```python
from build123d import *

# Parameters (mm, degrees)
BOSS_EXTRUDE2_DEPTH     = 500
SKETCH3_W               = 250
SKETCH3_H               = 50
CUT_EXTRUDE1_DEPTH      = 6
SKETCH5_W               = 50
SKETCH5_H               = 25
BOSS_EXTRUDE3_DEPTH     = 5
SKETCH7_W               = 50
SKETCH7_H               = 25
BOSS_EXTRUDE4_DEPTH     = 5
SKETCH8_R               = 2.5
CUT_EXTRUDE4_DEPTH      = 256
CUT_EXTRUDE4_DEPTH_BACK = 6
SKETCH11_R              = 5
BOSS_EXTRUDE15_DEPTH    = 250
BOSS_EXTRUDE16_DEPTH    = 10
BOSS_EXTRUDE17_DEPTH    = 10
CUT_EXTRUDE5_START      = -17
SKETCH30_R              = 2.5
CUT_EXTRUDE5_DEPTH      = 306.484848098
SKETCH31_R              = 2.5
CUT_EXTRUDE6_DEPTH      = 17


with BuildPart() as part:
    # Sketch2 → Boss-Extrude2 (new body)
    with BuildSketch(Plane.XY):
        Polygon((-130, 0), (130, 0), (130, 80), (115, 80), (115, 75), (125, 75), (125, 5), (-125, 5), (-125, 75), (-115, 75), (-115, 80), (-130, 80), align=None)
    extrude(amount=BOSS_EXTRUDE2_DEPTH)

    # Sketch3 → Cut-Extrude1 (cut, through all)
    with BuildSketch(Plane(origin=(0, 5, 0), x_dir=(1, 0, 0), z_dir=(0, 1, 0))):
        with Locations((0, -475)):
            Rectangle(SKETCH3_W, SKETCH3_H)
    extrude(amount=-CUT_EXTRUDE1_DEPTH, mode=Mode.SUBTRACT)

    # Sketch5 → Boss-Extrude3 (add)
    with BuildSketch(Plane.ZY.offset(-125)):
        with Locations((475, -12.5)):
            Rectangle(SKETCH5_W, SKETCH5_H)
    extrude(amount=-BOSS_EXTRUDE3_DEPTH)

    # Sketch7 → Boss-Extrude4 (add)
    with BuildSketch(Plane(origin=(-125, 0, 0), x_dir=(0, 0, -1), z_dir=(1, 0, 0))):
        with Locations((-475, -12.5)):
            Rectangle(SKETCH7_W, SKETCH7_H)
    extrude(amount=-BOSS_EXTRUDE4_DEPTH)

    # Sketch8 → Cut-Extrude4 (cut, two sides)
    with BuildSketch(Plane.ZY.offset(-125)) as cut_extrude4_sk:
        with Locations((470, 2.5)):
            Circle(SKETCH8_R)
    extrude(amount=CUT_EXTRUDE4_DEPTH, mode=Mode.SUBTRACT)
    extrude(cut_extrude4_sk.sketch, amount=-CUT_EXTRUDE4_DEPTH_BACK, mode=Mode.SUBTRACT)

    # Sketch11 → Boss-Extrude15 (add)
    with BuildSketch(Plane.ZY.offset(-125)):
        with Locations((480, 65)):
            Circle(SKETCH11_R)
    extrude(amount=BOSS_EXTRUDE15_DEPTH)

    # Sketch27 → Boss-Extrude16 (add)
    with BuildSketch(Plane(origin=(130, 0, 0), x_dir=(0, 0, -1), z_dir=(1, 0, 0))):
        Polygon((-20, 0), (-2.121320344, -17.878679656), (-4.242640687, -20), (-24.242640687, 0), align=None)
        Polygon((-39.798989873, 0), (-12.02081528, -27.778174593), (-14.142135624, -29.899494937), (-44.04163056, 0), align=None)
    boss_extrude16 = extrude(amount=-BOSS_EXTRUDE16_DEPTH)

    # Mirror1: Boss-Extrude16 across plane
    add(boss_extrude16.mirror(Plane.ZY))

    # Sketch29 → Boss-Extrude17 (add)
    with BuildSketch(Plane(origin=(130, 0, 0), x_dir=(0, 0, -1), z_dir=(1, 0, 0))):
        Polygon((-400, 0), (-420, -20), (-417.878679656, -22.121320344), (-395.757359313, 0), align=None)
        Polygon((-380.201010127, 0), (-410.100505063, -29.899494937), (-407.97918472, -32.02081528), (-375.95836944, 0), align=None)
    boss_extrude17 = extrude(amount=-BOSS_EXTRUDE17_DEPTH)

    # Mirror2: Boss-Extrude17 across plane
    add(boss_extrude17.mirror(Plane.ZY))

    # Sketch30 → Cut-Extrude5 (cut)
    with BuildSketch(Plane(origin=(0, 187.97918472, 187.97918472), x_dir=(1, 0, 0), z_dir=(0, -0.707106781, -0.707106781)).offset(CUT_EXTRUDE5_START)):
        with Locations((125, 306.126983722)):
            Circle(SKETCH30_R)
    cut_extrude5 = extrude(amount=CUT_EXTRUDE5_DEPTH, mode=Mode.SUBTRACT)

    # Mirror3: Cut-Extrude5 across plane
    add(cut_extrude5.mirror(Plane.ZY), mode=Mode.SUBTRACT)

    # Sketch31 → Cut-Extrude6 (cut)
    with BuildSketch(Plane(origin=(0, -22.02081528, 22.02081528), x_dir=(1, 0, 0), z_dir=(0, -0.707106781, 0.707106781))):
        with Locations((125, -6.142135624)):
            Circle(SKETCH31_R)
    cut_extrude6 = extrude(amount=-CUT_EXTRUDE6_DEPTH, mode=Mode.SUBTRACT)

    # Mirror5: Cut-Extrude6 across plane
    add(cut_extrude6.mirror(Plane.ZY), mode=Mode.SUBTRACT)


solid = part.part
```
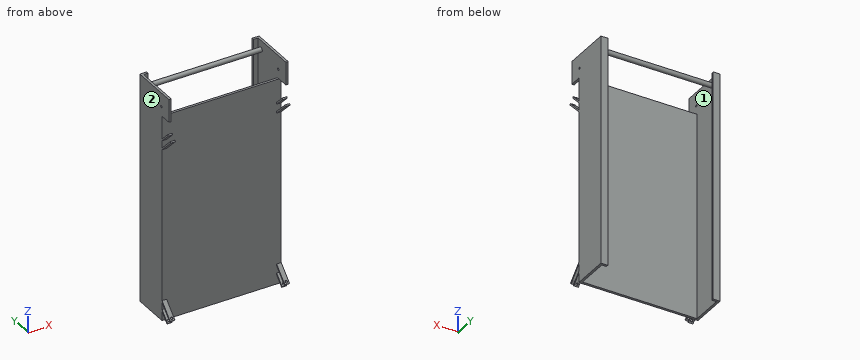
Verification items for the finished model (mm, model axes). Face numbers are marked on the shaded views. Coordinates: 2 decimals unless noted, no trailing zeros. Order: outer loops, then holes, each group sorted by start corner. A loop starts at its lowest first (then second) coordinate and runs counter-clockwise, first axis right, second up. Notation, with made-up numbers: (88.25, 40) - (145.25, 40) arc R18 cw to (145.25, 48) - close; hole circle Ø3 at (62, 52.5). An arc over 180 degrees is marked (long way). Return JSON: item names as keys, results as strings.
(1) Go/stop test with flat-tipped pins: pin 1 (16 mm diameter, centred on y = -17.5, z = 387, fed in from -X); pin 2 (4 mm diameter, centred on x = -128, z = 476.5, fed in from -Y); pin 3 (3 mm diameter, centred on x = -121, z = 282.5, fed in from -Y); pin 4 (4 mm diameter, centred on x = -127, y = -13, fed in from -Z). Record where each tip stops, or that it passes through.
Filled sheet:
{"pin 1": "stops at x = -130", "pin 2": "stops at y = -25", "pin 3": "stops at y = 0", "pin 4": "stops at z = 5.03"}
(2) Section check A-A, the plane y = 48. Record the cut outline in (x, z), and give its area (3 significant figures).
Filled sheet:
{"outline": "(-130, 0) - (-125, 0) - (-125, 500) - (-130, 500) - close; (125, 0) - (130, 0) - (130, 500) - (125, 500) - close", "area": "5,000 mm^2"}
(3) Thickness scan on line 1 along X through (y, z) = (19, 354.5); line 2 along Z through (x, y) = (127, 2); line 3 along Z through (x, y) = (-126.3, 2.5). Record the ranges inside material, lowest first.
Filled sheet:
{"line 1": "x = -130 to -125, 125 to 130", "line 2": "z = 0 to 467.55, 472.45 to 500", "line 3": "z = 0 to 467.5, 472.5 to 500"}
(4) Section check D-D, the plane z = 336. Record the cut outline in (x, y).
Filled sheet:
{"outline": "(-130, 0) - (130, 0) - (130, 80) - (115, 80) - (115, 75) - (125, 75) - (125, 5) - (-125, 5) - (-125, 75) - (-115, 75) - (-115, 80) - (-130, 80) - close"}
(5) Section check C-C, the plane z = 461. Record the cut outline in (x, y).
Filled sheet:
{"outline": "(-130, -25) - (-125, -25) - (-125, 75) - (-115, 75) - (-115, 80) - (-130, 80) - close; (115, 75) - (125, 75) - (125, -25) - (130, -25) - (130, 80) - (115, 80) - close"}
(6) Mould release check, pull along Y, two halves, no side actions. Record for the marked faces 1 and 2: pulls with the +Y half, pulls with the -Y half, needs draft (parallel to the pull), parting line crosses it, or undercut.
Filled sheet:
{"face 1": "undercut", "face 2": "needs draft"}
(7) Section check B-B, the plane x = 12.5. Record the cut outline in (y, z).
Filled sheet:
{"outline": "(0, 0) - (5, 0) - (5, 450) - (0, 450) - close; circle Ø10 at (65, 480)"}
